```python
from build123d import *

# Parameters (mm, degrees)
F0_W     = 37.211
F0_H     = 24.511
F1_DEPTH = 68.58
F2_T     = -1.5875
F3_R     = 4.445
F4_DEPTH = 1.5875
F5_R     = 1.27


with BuildPart() as f1:
    # F0 (on Top) → F1 (new body)
    with BuildSketch(Plane.XY):
        Rectangle(F0_W, F0_H)
    extrude(amount=F1_DEPTH)

    # F2
    f2_openings = [f1.faces().sort_by_distance(p)[0] for p in [
        (0, 12.2555, 34.29),
    ]]
    offset(amount=F2_T, openings=f2_openings)

    # F3 (on face) → F4 (cut)
    with BuildSketch(Plane.XY.offset(68.58)):
        with Locations((12.573, 0)):
            Circle(F3_R)
    extrude(amount=-F4_DEPTH, mode=Mode.SUBTRACT)

    # F5
    f5_edges = [f1.edges().sort_by_distance(p)[0] for p in [
        (-18.6055, 12.2555, 34.29),
        (0, 12.2555, 68.58),
        (18.6055, 12.2555, 34.29),
        (0, 12.2555, 0),
    ]]
    fillet(f5_edges, radius=F5_R)


solid = f1.part
```
Work out the finished part from the listing and answer in its coordinate system (mm). A direction names the side the tool comes from. Give positions to 0.01 mm unless a question says otherwise; leave off trailing zeros. Order: outer loops, then holes, each group sorted by start corner. A loop starts at its lowest first (then second) coordinate and runs counter-clockwise, first axis right, second up. Notation, with made-up numbers: (-22.5, 72.5) - (11.5, 72.5) arc R36 cw to (11.5, 110.5) - close; hole circle Ø5 at (63, 26). An arc over 180 degrees is marked (long way). One line per item, written item: value. Start each with the question number.
1. Which of the six approach directions +Z, -Z, +X, -X, +Y, -Y give full straight-line access (tool end or side, diameter ignored) to faces 4 (the face through (-18.606, -1, 34)), 5 (the face through (0, -10.668, 34))?
2. For a pull along X with two mould halves and no side action, classify faces 1 (the face through (8.132, 0.195, 67.797)), 2 (the face through (0, 0, 0)), 3 (the face through (18.606, -1, 34)) as released by +X, released by -X, zero draft, split by the parting line, or undercut.
3. Section D-D, the plane y = -2.5 is taken. Write down the section's boundary in (x, z).
4. Consider line 1 (X direction, y = 2, z = 28); line 2 (Z direction, x = -7, y = -3.25); line 3 (Z direction, x = 13, y = -4.25). Determine where each line is inside the solid, lowest interval first.
5. Section C-C, the plane y = 0.75 is taken. Write down the section's boundary in (x, z).
6. This flat-tipped pin is pushed along its axis until it touches: pin 1 Ø10 at (x, z) = (-8, 30.5) entering from +Y. Where does it stop, or does it pass through?
7. Section A-A, the plane y = 9.5 is taken. Write down the section's boundary in (x, z).
8. Section B-B, the plane z = 19.5 is taken. Write down the section's boundary in (x, y).
Filled sheet:
1. face 4: +Z, -Z, -X, +Y, -Y
1. face 5: +Y
2. face 1: undercut
2. face 2: zero draft
2. face 3: released by +X
3. outline: (-18.61, 0) - (18.61, 0) - (18.61, 68.58) - (16.25, 68.58) - (16.25, 66.99) - (17.02, 66.99) - (17.02, 1.59) - (-17.02, 1.59) - (-17.02, 66.99) - (8.9, 66.99) - (8.9, 68.58) - (-18.61, 68.58) - close
4. line 1: -18.61 to -17.02, 17.02 to 18.61
4. line 2: 0 to 1.59, 66.99 to 68.58
4. line 3: 0 to 1.59
5. outline: (-18.61, 0) - (18.61, 0) - (18.61, 68.58) - (16.95, 68.58) - (16.95, 66.99) - (17.02, 66.99) - (17.02, 1.59) - (-17.02, 1.59) - (-17.02, 66.99) - (8.19, 66.99) - (8.19, 68.58) - (-18.61, 68.58) - close
6. pin 1: y = -10.67
7. outline: (-18.61, 0) - (18.61, 0) - (18.61, 68.58) - (-18.61, 68.58) - close; hole (-17.02, 1.59) - (17.02, 1.59) - (17.02, 66.99) - (-17.02, 66.99) - close
8. outline: (-18.61, -12.26) - (18.61, -12.26) - (18.61, 10.99) arc R1.27 ccw to (17.34, 12.26) - (17.02, 12.26) - (17.02, -10.67) - (-17.02, -10.67) - (-17.02, 12.26) - (-17.34, 12.26) arc R1.27 ccw to (-18.61, 10.99) - close
